Autodesk Inventor part; units mm, degrees
ref_plane "YZ Plane" through (0, 0, 0) normal (1, 0, 0) x (0, 1, 0)
ref_plane "XZ Plane" through (0, 0, 0) normal (0, 1, 0) x (-1, 0, 0)
ref_plane "XY Plane" through (0, 0, 0) normal (0, 0, 1) x (1, 0, 0)
sketch "Sketch1" plane through (0, 0, 0) normal (0, 0, 1) x (1, 0, 0)
  circle A0 centre (0, 0) radius 6.825
  dimension "d0" = 13.65
extrude "Extrusion1" add sketch "Sketch1" along normal blind 6.4
sketch "Sketch2" plane through (0, 0, 6.4) normal (0, 0, 1) x (1, 0, 0)
  circle A0 centre (-4.05, 0) radius 1.2
  circle A1 centre (4.05, 0) radius 1.2
  circle A2 centre (0, -4.05) radius 1.2
  circle A3 centre (0, 0) radius 4.05 construction
  dimension "d3" = 2.4
  dimension "d4" = 2.4
  dimension "d5" = 2.4
  dimension "d6" = 8.1
extrude "Extrusion2" add sketch "Sketch2" along normal blind 12
fillet "Fillet1" radius 1.15 3 edges at (-5.25, 0, 18.4) (2.85, 0, 18.4) (-1.2, -4.05, 18.4)
sketch "Sketch3" plane through (0, 0, 0) normal (0, 0, -1) x (-1, 0, 0)
  circle A0 centre (-4.05, 0) radius 1.2
  circle A1 centre (4.05, 0) radius 1.2
  circle A2 centre (0, -4.05) radius 1.2
  point P0 (0, 0)
extrude "Extrusion3" add sketch "Sketch3" along normal blind 4
sketch "Sketch4" plane through (0, 0, 6.4) normal (0, 0, 1) x (1, 0, 0)
  line L0 (-1, 6.825) -> (1, 6.825)
  line L1 (1, 6.825) -> (1, 4.325)
  line L2 (1, 4.325) -> (-1, 4.325)
  line L3 (-1, 4.325) -> (-1, 6.825)
  circle A0 centre (0, 0) radius 6.825
  point P0 (0, 4.325)
  point P1 (0, 6.825)
  point P2 (1, 6.7513)
  point P3 (-1, 6.7513)
  dimension "d12" = 2
  dimension "d13" = 2.5
extrude "Extrusion4" cut sketch "Sketch4" against normal through all contours A0 L1 L2 L3 picked at (0, 5.1583)
sketch "Sketch5" plane through (0, 0, 6.4) normal (0, 0, 1) x (1, 0, 0)
  arc A0 (-1, 6.7513) -> (1, 6.7513) centre (0, 0) ccw
  arc A1 (-1.1465, 7.7406) -> (1.1465, 7.7406) centre (0, 0) ccw
  arc A2 (-1, 6.7513) -> (1, 6.7513) centre (0, 0) ccw
  line L0 (-1, -6.7513) -> (-1, -7.7608)
  line L1 (1, -6.7513) -> (1, -7.7608)
  dimension "d16" = 1
  dimension "d17" = 1
  dimension "d18" = 1
extrude "Extrusion5" add sketch "Sketch5" against normal up to surface (6.4 mm away)
pattern_circular "Circular Pattern1" count 2 over 120 about axis through (0, 0, 0) along (0, 0, -1) of "Extrusion5"
properties part number "NeutrikXLR" material "ABS Plastic"
Could you check a few things on this model? Use its own coordinates, in mm. A direction names the side the tool comes from. Coordinates: 2 decimals unless noted, no trailing zeros. Order: outer loops, then holes, each group sorted by start corner. A loop starts at its lowest first (then second) coordinate and runs counter-clockwise, first axis right, second up.
Q1. Which directions (+Z, -Z, +X, -X, +Y, -Y) give clear straight access to the entire face, cutting with the end or side of a thin tool? Please do faces 1 (the cylindrical face through (-0.26, -2.88, 11.75)), 2 (the flat face through (0, 0, 0)), 3 (the flat face through (1, -7, 3)), 4 (the flat face through (-1, 6, 3)).
Q2. Please list where these lines run through material, in increasing order: L1, parallel to Z at x = 3, y = -1; L2, parallel to X at y = 0.75, z = -0.75; L3, parallel to Y at x = -4, z = 16.
Q3. Suppose I cut it at C-C on z = 1. Please give me the cut outline in (x, y) (3 decimals), and give its area (3 significant figures).
Q4. Suppose I cut it at D-D on x = 2.5. Please give me the cut outline in (y, z).
Q5. Will these pins go through, and if not, where does the flat tip stop? pin 1 (4 mm diameter, centred on x = 5, z = 9.5, fed in from -Y); pin 2 (0.6 mm diameter, centred on x = -0.5, z = 4.5, fed in from +Y) (3 decimals); pin 3 (4 mm diameter, centred on y = -5.5, z = 12.5, fed in from +X).
Q6. Suppose I cut it at A-A on z = 11. Please give me the cut outline in (x, y).
Q7. Thinking about a two-plate mould opening in Y: for faces 5 (the flat face through (1, 6, 3)), 6 (the cylindrical face through (2.85, -0.05, 11.75)), 7 (the flat face through (-6.78, 2.76, 3.24)), 8 (the cylindrical face through (-5.867, -3.487, 3.155)), which applies, released by +Y, released by -Y, zero draft, split by the parting line, or undercut?
Q8. Suppose I cut it at B-B on y = -7. Please give me the cut outline in (x, z).
Answer:
1. face 1: +Z
1. face 2: -Z
1. face 3: +Z, -Z, +X, -Y
1. face 4: +Z, -Z, +Y
2. L1: z = 0 to 6.4
2. L2: x = -4.99 to -3.11, 3.11 to 4.99
2. L3: y = -1.2 to 1.2
3. outline: (-7.221, 3.014) - (-6.347, 2.51) arc R6.825 ccw to (-1, -6.751) - (-1, -7.761) arc R7.825 ccw to (1, -7.761) - (1, -6.751) arc R6.825 ccw to (1, 6.751) - (1, 4.325) - (-1, 4.325) - (-1, 6.751) arc R6.825 ccw to (-5.347, 4.242) - (-6.221, 4.746) arc R7.825 ccw to start
3. area: 145 mm2
4. outline: (-6.35, 0) - (6.35, 0) - (6.35, 6.4) - (-6.35, 6.4) - close
5. pin 1: stops at y = -1.2
5. pin 2: stops at y = 4.325
5. pin 3: stops at x = 1.2
6. outline: circle Ø2.4 at (-4.05, 0); circle Ø2.4 at (0, -4.05); circle Ø2.4 at (4.05, 0)
7. face 5: zero draft
7. face 6: split by the parting line
7. face 7: undercut
7. face 8: undercut
8. outline: (-1, 0) - (1, 0) - (1, 6.4) - (-1, 6.4) - close
